Read the model definition and answer for the solid it produces. Units are mm, in the model's axes. A direction names the side the tool comes from. Round coordinates to 2 decimals unless told otherwise and drop trailing zeros. Order: outer loops, then holes, each group sorted by start corner. A loop starts at its lowest first (then second) coordinate and runs counter-clockwise, first axis right, second up. Notation, with made-up numbers: M 39.25,-22 L 46.25,-22 A24 ccw 46.25,17 Z; hole C -4,35 d10. An arc over 180 degrees is marked long. Answer as CSV lines item,"result".
```python
from build123d import *

# Parameters (mm, degrees)
F2_R     = 19.05
F3_DEPTH = 25.4
F4_SIZE  = 1.5875


with BuildPart() as f1:
    # F0 (on Right) → F1 (revolve)
    with BuildSketch(Plane.YZ):
        Polygon((-25.4, 19.05), (0, 19.05), (25.4, 19.05), (25.4, 38.1), (6.35, 38.1), (6.35, 107.95), (12.7, 107.95), (12.7, 133.35), (0, 133.35), (-12.7, 133.35), (-12.7, 107.95), (-6.35, 107.95), (-6.35, 38.1), (-25.4, 38.1), align=None)
    revolve(axis=Axis((0, 38.140107, 0), (0, 1, 0)))

    # F2 (on face) → F3 (cut)
    with BuildSketch(Plane.XZ.offset(6.35)):
        with Locations((73.57686, 0)):
            Circle(F2_R)
        with Locations((0, -73.57686)):
            Circle(F2_R)
        with Locations((-73.57686, 0)):
            Circle(F2_R)
        with BuildLine():
            ThreePointArc((19.05, 73.57686), (-13.470384, 87.047244), (0, 54.52686))
            ThreePointArc((0, 54.52686), (13.470384, 60.106476), (19.05, 73.57686))
        make_face()
    extrude(amount=-F3_DEPTH, mode=Mode.SUBTRACT)

    # F4
    f4_edges = [f1.edges().sort_by_distance(p)[0] for p in [
        (0, -25.4, -19.05),
        (0, -25.4, -38.1),
    ]]
    chamfer(f4_edges, length=F4_SIZE)


solid = f1.part
```
Item 1: Flat-ended cylindrical pins translate along their axes: pin 1 (10 mm diameter, centred on x = -15, y = 10.5, fed in from -Z); pin 2 (8 mm diameter, centred on y = -4, z = -27, fed in from +X); pin 3 (2 mm diameter, centred on x = 24, y = 8.5, fed in from -Z). Find the tip coordinate at first contact, or state that the pin passes through.
Ans:
pin 1,"z = -132.97"
pin 2,"x = 131.35"
pin 3,"z = -131.35"
Item 2: Determine the mould class of faces 4 (the face through (40.055, -0.178, 127.192)), 5 (the face through (-108, -12.7, -11)), 6 (the face through (91.747, -0.089, 5.722)) for opening direction Z: +Z half, -Z half, draft (parallel to the pull), parting line (faces both ways), or undercut.
Ans:
face 4,"parting line"
face 5,"draft"
face 6,"undercut"
Item 3: Find the intervals of material crossed by probe 1 along Z at (x, y) = (1, -13.5); probe 2 along Z at (x, y) = (-20.5, -12.5); probe 3 along Z at (x, y) = (5.5, 2), in increasing order. Write a range as [from, to].
Ans:
probe 1,"[-38.09, -19.02], [19.02, 38.09]"
probe 2,"[-131.76, -105.99], [-32.11, 32.11], [105.99, 131.76]"
probe 3,"[-133.24, -91.82], [-55.34, -18.24], [18.24, 55.34], [91.82, 133.24]"
Item 4: A tool of negligible diameter and unlimited length cuts with its end or side. For faces 1 (the face through (72.96, 9.57, -79.56)), 2 (the face through (-92.61, -0.09, 0.84)), 3 (the face through (-23.183, -15.203, -30.235)), from which of +Z, -Z, +X, -X, +Y, -Y can it reach the whole face along a straight path? Write none if from no direction.
Ans:
face 1,"+Y"
face 2,"+Y, -Y"
face 3,"-Y"
Item 5: A cutting plane is placed at B-B, the plane z = 63. Determine the outline of the cut face in (x, y).
Ans:
outline,"M -117.53,-12.7 L -87.66,-12.7 L -87.66,-6.35 L -15.84,-6.35 L -15.84,6.35 L -87.66,6.35 L -87.66,12.7 L -117.53,12.7 Z; M 15.84,-6.35 L 87.66,-6.35 L 87.66,-12.7 L 117.53,-12.7 L 117.53,12.7 L 87.66,12.7 L 87.66,6.35 L 15.84,6.35 Z"
Item 6: A cutting plane is placed at C-C, the plane y = -20. Determine the outline of the cut face in (x, z).
Ans:
outline,"C 0,0 d76.2; hole C 0,0 d38.1"
Item 7: A cutting plane is placed at A-A, the plane x = 83. Determine the outline of the cut face in (y, z), and give its area (3 significant figures).
Ans:
outline,"M -12.7,-104.37 L 12.7,-104.37 L 12.7,-69.02 L 6.35,-69.02 L 6.35,-16.56 L -6.35,-16.56 L -6.35,-69.02 L -12.7,-69.02 Z; M -12.7,69.02 L -6.35,69.02 L -6.35,16.56 L 6.35,16.56 L 6.35,69.02 L 12.7,69.02 L 12.7,104.37 L -12.7,104.37 Z"
area,"3,130 mm2"
Item 8: A cutting plane is placed at D-D, the plane x = 46.5. Determine the outline of the cut face in (y, z), and give its area (3 significant figures).
Ans:
outline,"M -12.7,-124.98 L 12.7,-124.98 L 12.7,-97.42 L 6.35,-97.42 L 6.35,97.42 L 12.7,97.42 L 12.7,124.98 L -12.7,124.98 L -12.7,97.42 L -6.35,97.42 L -6.35,-97.42 L -12.7,-97.42 Z"
area,"3,870 mm2"
